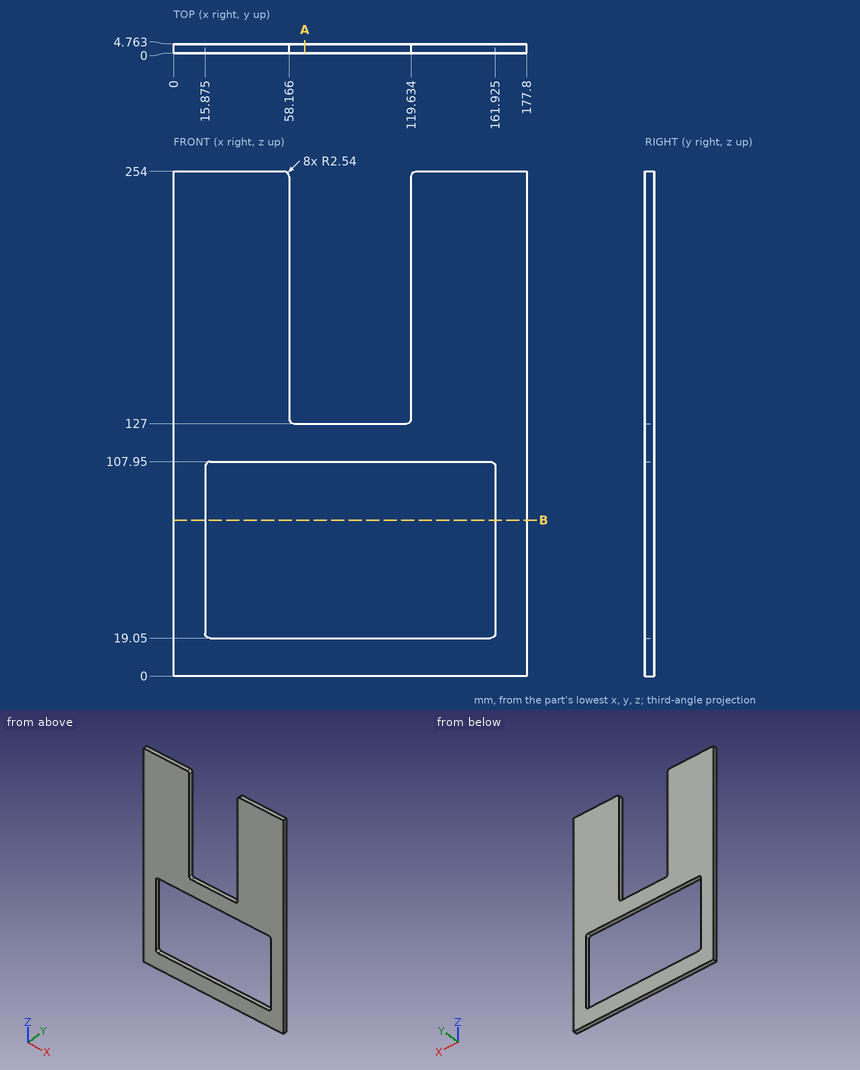
Verification items for this drawing (mm, ordinates from the low corner). Coordinates: 2 decimals unless noted, no trailing zeros. Order: outer loops, then holes, each group sorted by start corner. A loop starts at its lowest first (then second) coordinate and runs counter-clockwise, first axis right, second up. Notation, with made-up numbers: M -17,21.25 L 29,21.25 A10 ccw 29,34.25 Z; hole C -16,0 d4. An arc over 180 degrees is marked long. Use CSV: the item, a comma, the result in double quotes.
Item 1: Gauge pin test, flat end, axial feed: pin 1 Ø1.4 at (x, y) = (82.5, 3) entering from +Z. Record the tip position at first contact, or that the pin passes through.
Returned:
pin 1,"stops at z = 127"
Item 2: Cross-section at B-B on z = 78.5. Record the cut outline in (x, y) (1 decimal).
Returned:
outline,"M 0,0 L 15.9,0 L 15.9,4.8 L 0,4.8 Z; M 161.9,0 L 177.8,0 L 177.8,4.8 L 161.9,4.8 Z"
Item 3: Cross-section at A-A on x = 66. Record the cut outline in (y, z).
Returned:
outline,"M 0,0 L 4.76,0 L 4.76,19.05 L 0,19.05 Z; M 0,107.95 L 4.76,107.95 L 4.76,127 L 0,127 Z"
Item 4: Thickness scan on line 1 along X through (y, z) = (1.75, 172) (1 decimal); line 2 along Z through (x, y) = (34, 4.4); line 3 along X through (y, z) = (1.3, 55.5) (1 decimal). Record the ranges inside material, lowest first.
Returned:
line 1,"x = 0 to 58.2, 119.6 to 177.8"
line 2,"z = 0 to 19.05, 107.95 to 254"
line 3,"x = 0 to 15.9, 161.9 to 177.8"
